Can you work these out from the model? Positions are in its coordinate system, mm. A direction names the side the tool comes from. Give positions to 0.01 mm unless a question says otherwise; leave off trailing zeros. Order: outer loops, then holes, each group sorted by start corner. A loop starts at its lowest first (then second) coordinate and runs counter-clockwise, first axis right, second up. Notation, with made-up numbers: (64.25, 75) - (121.25, 75) arc R21 cw to (121.25, 80) - close; hole circle Ø6 at (56, 60). An arc over 180 degrees is marked (long way). Use one line per item in the form item = value. Start each with the question number.
1) Suppose I cut it at A-A, the plane y = 88.9. Write out the boundary of the cut face in (x, z), and give its area (3 significant figures).
2) Please list where these lines run through material, in increasing order: probe 1 along Y at (x, z) = (-322, 1); probe 2 along Y at (x, z) = (-210.5, 3.25); probe 3 along Y at (x, z) = (-369.5, 4.5).
3) Suppose I cut it at B-B, the plane z = 4. State how many separate pieces and enclosed holes the cut face has, and give its area (3 significant figures).
4) We'd pull the mould along Y, two halves only. Please class faces 1 (the flat face through (-41.61, 35.26, 3.13)), 2 (the flat face through (-417.563, 31.306, 3.131)), 3 (the flat face through (-326.913, 31.959, 3.131)), 4 (the flat face through (-215, 60, 6.35)): released by +Y, released by -Y, zero draft, split by the parting line, or undercut.
5) For pin 1 (1.9 mm diameter, centred on x = -174, z = 2, fed in from -Y); pin 2 (1.9 mm diameter, centred on x = -35.5, z = 2, fed in from -Y); pin 3 (3 mm diameter, centred on y = 37, z = 4.5, fed in from -X), each with a flat end and sliding along its axis, tell me the tip position at first contact or that it passes through.
6) Which directions (+Z, -Z, +X, -X, +Y, -Y) give clear straight access to the entire face, cutting with the end or side of a thin tool? Please do faces 5 (the flat face through (-346.41, 35.26, 3.13)), 6 (the flat face through (-215, 60, 0)).
```python
from build123d import *

# Parameters (mm, degrees)
MODEL_R             = 4
BOSS_EXTRUDE1_DEPTH = 6.35
SKETCH1_W           = 10.16
SKETCH1_H           = 6.35
SKETCH1_W_2         = 436.88
BOSS_EXTRUDE2_DEPTH = 6.35
SKETCH2_W           = 6.35
SKETCH2_H           = 10.16
BOSS_EXTRUDE3_DEPTH = 6.35
SKETCH2_3_W         = 6.35
SKETCH2_3_H         = 6.35
SKETCH2_3_H_2       = 12.7
CUT_EXTRUDE1_DEPTH  = 6.35
SKETCH3_W           = 12.986644794
SKETCH3_H           = 59.111624581
BOSS_EXTRUDE4_DEPTH = 6.35
BOSS_EXTRUDE6_DEPTH = 6.35


with BuildPart() as part:
    # Model → Boss-Extrude1 (new body)
    with BuildSketch(Plane.XY):
        Polygon((-398.78, 0), (-436.88, 63.5), (-436.88, 95.25), (0, 95.25), (0, 0), align=None)
        with Locations((-172.466, 88.9)):
            Circle(MODEL_R, mode=Mode.SUBTRACT)
        with Locations((-339.23478, 68.423282)):
            Circle(MODEL_R, mode=Mode.SUBTRACT)
        with BuildLine():
            Line((-306.628052638, 15.624984002), (-306.628052638, 51.149330332))
            ThreePointArc((-306.628052638, 51.149330332), (-307.372001413, 52.945381557), (-309.168052638, 53.689330332))
            Line((-309.168052638, 53.689330332), (-340.406029433, 53.689330332))
            ThreePointArc((-340.406029433, 53.689330332), (-342.720322456, 52.196062295), (-342.31346603, 49.472045137))
            Line((-342.31346603, 49.472045137), (-311.075489235, 13.947698807))
            ThreePointArc((-311.075489235, 13.947698807), (-308.271751616, 13.248380443), (-306.628052638, 15.624984002))
        make_face(mode=Mode.SUBTRACT)
        with BuildLine():
            Line((-171.232102448, 6.35), (-215.9, 6.35))
            ThreePointArc((-215.9, 6.35), (-220.390128061, 8.209871939), (-222.25, 12.7))
            Line((-222.25, 12.7), (-222.25, 57.367897552))
            ThreePointArc((-222.25, 57.367897552), (-220.682015918, 59.714551564), (-217.913948776, 59.163948776))
            Line((-217.913948776, 59.163948776), (-169.436051224, 10.686051224))
            ThreePointArc((-169.436051224, 10.686051224), (-168.885448436, 7.917984082), (-171.232102448, 6.35))
        make_face(mode=Mode.SUBTRACT)
        with BuildLine():
            Line((-234.95, 57.367897552), (-234.95, 12.7))
            ThreePointArc((-234.95, 12.7), (-236.809871939, 8.209871939), (-241.3, 6.35))
            Line((-241.3, 6.35), (-285.967897552, 6.35))
            ThreePointArc((-285.967897552, 6.35), (-288.314551564, 7.917984082), (-287.763948776, 10.686051224))
            Line((-287.763948776, 10.686051224), (-239.286051224, 59.163948776))
            ThreePointArc((-239.286051224, 59.163948776), (-236.517984082, 59.714551564), (-234.95, 57.367897552))
        make_face(mode=Mode.SUBTRACT)
        with BuildLine():
            Line((-294.113948776, 17.036051224), (-245.636051224, 65.513948776))
            ThreePointArc((-245.636051224, 65.513948776), (-245.085448436, 68.282015918), (-247.432102448, 69.85))
            Line((-247.432102448, 69.85), (-292.1, 69.85))
            ThreePointArc((-292.1, 69.85), (-296.590128061, 67.990128061), (-298.45, 63.5))
            Line((-298.45, 63.5), (-298.45, 18.832102448))
            ThreePointArc((-298.45, 18.832102448), (-296.882015918, 16.485448436), (-294.113948776, 17.036051224))
        make_face(mode=Mode.SUBTRACT)
        with BuildLine():
            Line((-323.632102448, 6.35), (-368.3, 6.35))
            ThreePointArc((-368.3, 6.35), (-372.790128061, 8.209871939), (-374.65, 12.7))
            Line((-374.65, 12.7), (-374.65, 57.367897552))
            ThreePointArc((-374.65, 57.367897552), (-373.082015918, 59.714551564), (-370.313948776, 59.163948776))
            Line((-370.313948776, 59.163948776), (-321.836051224, 10.686051224))
            ThreePointArc((-321.836051224, 10.686051224), (-321.285448436, 7.917984082), (-323.632102448, 6.35))
        make_face(mode=Mode.SUBTRACT)
        with BuildLine():
            Line((-18.832102448, 6.35), (-63.5, 6.35))
            ThreePointArc((-63.5, 6.35), (-67.990128061, 8.209871939), (-69.85, 12.7))
            Line((-69.85, 12.7), (-69.85, 57.367897552))
            ThreePointArc((-69.85, 57.367897552), (-68.282015918, 59.714551564), (-65.513948776, 59.163948776))
            Line((-65.513948776, 59.163948776), (-17.036051224, 10.686051224))
            ThreePointArc((-17.036051224, 10.686051224), (-16.485448436, 7.917984082), (-18.832102448, 6.35))
        make_face(mode=Mode.SUBTRACT)
        with BuildLine():
            Line((-82.55, 57.367897552), (-82.55, 12.7))
            ThreePointArc((-82.55, 12.7), (-84.409871939, 8.209871939), (-88.9, 6.35))
            Line((-88.9, 6.35), (-133.567897552, 6.35))
            ThreePointArc((-133.567897552, 6.35), (-135.914551564, 7.917984082), (-135.363948776, 10.686051224))
            Line((-135.363948776, 10.686051224), (-86.886051224, 59.163948776))
            ThreePointArc((-86.886051224, 59.163948776), (-84.117984082, 59.714551564), (-82.55, 57.367897552))
        make_face(mode=Mode.SUBTRACT)
        with BuildLine():
            Line((-93.236051224, 65.513948776), (-141.713948776, 17.036051224))
            ThreePointArc((-141.713948776, 17.036051224), (-144.482015918, 16.485448436), (-146.05, 18.832102448))
            Line((-146.05, 18.832102448), (-146.05, 63.5))
            ThreePointArc((-146.05, 63.5), (-144.190128061, 67.990128061), (-139.7, 69.85))
            Line((-139.7, 69.85), (-95.032102448, 69.85))
            ThreePointArc((-95.032102448, 69.85), (-92.685448436, 68.282015918), (-93.236051224, 65.513948776))
        make_face(mode=Mode.SUBTRACT)
        with BuildLine():
            Line((-163.086051224, 17.036051224), (-211.563948776, 65.513948776))
            ThreePointArc((-211.563948776, 65.513948776), (-212.114551564, 68.282015918), (-209.767897552, 69.85))
            Line((-209.767897552, 69.85), (-165.1, 69.85))
            ThreePointArc((-165.1, 69.85), (-160.609871939, 67.990128061), (-158.75, 63.5))
            Line((-158.75, 63.5), (-158.75, 18.832102448))
            ThreePointArc((-158.75, 18.832102448), (-160.317984082, 16.485448436), (-163.086051224, 17.036051224))
        make_face(mode=Mode.SUBTRACT)
        with BuildLine():
            Line((-6.35, 63.5), (-6.35, 18.832102448))
            ThreePointArc((-6.35, 18.832102448), (-7.917984082, 16.485448436), (-10.686051224, 17.036051224))
            Line((-10.686051224, 17.036051224), (-59.163948776, 65.513948776))
            ThreePointArc((-59.163948776, 65.513948776), (-59.714551564, 68.282015918), (-57.367897552, 69.85))
            Line((-57.367897552, 69.85), (-12.7, 69.85))
            ThreePointArc((-12.7, 69.85), (-8.209871939, 67.990128061), (-6.35, 63.5))
        make_face(mode=Mode.SUBTRACT)
    extrude(amount=BOSS_EXTRUDE1_DEPTH)

    # Sketch1 → Boss-Extrude2 (add)
    with BuildSketch(Plane.XY.offset(6.35)):
        with Locations((-75.565, -3.175)):
            Rectangle(SKETCH1_W, SKETCH1_H)
        with Locations((-151.13, -3.175)):
            Rectangle(SKETCH1_W, SKETCH1_H)
        with Locations((-227.965, -3.175)):
            Rectangle(SKETCH1_W, SKETCH1_H)
        with Locations((-303.53, -3.175)):
            Rectangle(SKETCH1_W, SKETCH1_H)
        with Locations((-373.38, -3.175)):
            Rectangle(SKETCH1_W, SKETCH1_H)
        with Locations((-218.44, 98.425)):
            Rectangle(SKETCH1_W_2, SKETCH1_H)
    extrude(amount=-BOSS_EXTRUDE2_DEPTH)

    # Sketch2 → Boss-Extrude3 (add)
    # profile 1 of 3: a face of its own
    with BuildSketch(Plane(origin=(0, 0, 0), x_dir=(-1, 0, 0), z_dir=(0, 0, -1))):
        Polygon((185.42, 39.37), (185.42, 69.85), (177.8, 69.85), (177.8, 63.5), (171.45, 63.5), (171.45, 69.85), (165.1, 69.85), (165.1, 19.05), align=None)
        with Locations((174.625, 38.1)):
            Rectangle(SKETCH2_W, SKETCH2_H, mode=Mode.SUBTRACT)
    # profile 2 of 3: a face of its own
    with BuildSketch(Plane(origin=(0, 0, 0), x_dir=(-1, 0, 0), z_dir=(0, 0, -1))):
        Polygon((185.42, 6.35), (185.42, 26.67), (171.45, 12.7), (177.8, 12.7), (177.8, 6.35), align=None)
    # profile 3 of 3: a face of its own
    with BuildSketch(Plane(origin=(0, 0, 0), x_dir=(-1, 0, 0), z_dir=(0, 0, -1))):
        with BuildLine():
            Line((171.45, 6.35), (171.45, 12.7))
            Line((171.45, 12.7), (169.436051224, 10.686051224))
            ThreePointArc((169.436051224, 10.686051224), (168.885448436, 7.917984082), (171.232102448, 6.35))
            Line((171.232102448, 6.35), (171.45, 6.35))
        make_face()
    extrude(amount=-BOSS_EXTRUDE3_DEPTH)

    # Sketch2<3> → Cut-Extrude1 (cut)
    with BuildSketch(Plane(origin=(0, 0, 0), x_dir=(-1, 0, 0), z_dir=(0, 0, -1))):
        with Locations((174.625, 73.025)):
            Rectangle(SKETCH2_3_W, SKETCH2_3_H)
        with Locations((174.625, 6.35)):
            Rectangle(SKETCH2_3_W, SKETCH2_3_H_2)
    extrude(amount=-CUT_EXTRUDE1_DEPTH, mode=Mode.SUBTRACT)

    # Sketch3 → Boss-Extrude4 (add)
    with BuildSketch(Plane(origin=(0, 0, 0), x_dir=(-1, 0, 0), z_dir=(0, 0, -1))):
        with Locations((160.895729101, 43.146846623)):
            Rectangle(SKETCH3_W, SKETCH3_H)
    extrude(amount=-BOSS_EXTRUDE4_DEPTH)

    # Sketch4 → Boss-Extrude6 (add)
    with BuildSketch(Plane.XY.offset(6.35)):
        with BuildLine():
            ThreePointArc((-187.96, 6.35), (-186.163948776, 7.093948776), (-185.42, 8.89))
            Line((-185.42, 8.89), (-185.42, 6.35))
            Line((-185.42, 6.35), (-187.96, 6.35))
        make_face()
        with BuildLine():
            Line((-185.42, 26.67), (-186.163948776, 27.413948776))
            ThreePointArc((-186.163948776, 27.413948776), (-185.613345987, 26.58991347), (-185.42, 25.617897552))
            Line((-185.42, 25.617897552), (-185.42, 26.67))
        make_face()
        with BuildLine():
            Line((-185.42, 45.502102448), (-185.42, 39.37))
            Line((-185.42, 39.37), (-189.756051224, 43.706051224))
            ThreePointArc((-189.756051224, 43.706051224), (-186.987984082, 43.155448436), (-185.42, 45.502102448))
        make_face()
        with BuildLine():
            Line((-187.96, 69.85), (-185.42, 69.85))
            Line((-185.42, 69.85), (-185.42, 67.31))
            ThreePointArc((-185.42, 67.31), (-186.163948776, 69.106051224), (-187.96, 69.85))
        make_face()
    extrude(amount=-BOSS_EXTRUDE6_DEPTH)


solid = part.part
```
Result sheet:
q1.outline = (-436.88, 0) - (-176.47, 0) - (-176.47, 6.35) - (-436.88, 6.35) - close; (-168.47, 0) - (0, 0) - (0, 6.35) - (-168.47, 6.35) - close
q1.area = 2,720 mm²
q2.probe_1 = 0 to 6.94, 10.85 to 26.37, 53.69 to 101.6
q2.probe_2 = 0 to 6.35, 51.75 to 64.45, 69.74 to 101.6
q2.probe_3 = -6.35 to 6.46, 58.35 to 101.6
q3.separate_pieces = 1
q3.enclosed_holes = 14
q3.area = 29,200 mm²
q4.face_1 = undercut
q4.face_2 = released by -Y
q4.face_3 = undercut
q4.face_4 = zero draft
q5.pin_1 = 12.7
q5.pin_2 = 0
q5.pin_3 = -421.88
q6.face_5 = +Z, -Z
q6.face_6 = -Z, +X, -X, +Y, -Y
